Geometry: see drawing. Coordinates: mm, zero at the bounding-box minimum. A direction names the side the tool comes from. Coordinates: 2 decimals unless noted, no trailing zeros. Write each loop counter-clockwise with the first axis right and the second up, starting at its lowest first coordinate (ties: lowest second). Pieces come first, ordered by that corner, then holes. Notation, with made-up numbers: (-25.5, 61.25) - (-11.5, 61.25) arc R25 ccw to (-11.5, 96.25) - close; hole circle Ø11 at (24, 67.25). An arc over 180 degrees is marked (long way). Use a Markdown table: item, result. Add a question column.
Q1. Section query A-A (z = 4). Return the cut outline in (x, y).
Q2. Set-up query: the marked faces 1, 2 and 3. Return all of +Z, -Z, +X, -X, +Y, -Y with unobstructed straight access to the full face (end or side cutting, diameter ignored); none if empty.
Q3. Section query B-B (x = 28.5). Return the cut outline in (y, z).
Q4. Pin query (flat end, axial travel): P1, Ø5, axis at x = 24.5, y = 9.5, coming from the -Z side; P2, Ø8, axis at y = 10.5, z = 8, coming from the -X side; P3, Ø16, axis at x = 19.5, z = 27.5, coming from the +Y side. Return the tip coordinate at first contact, or that it passes through.
Q5. Section query C-C (x = 44). Return the cut outline in (y, z).
Q6. Section query D-D (z = 30). Return the cut outline in (x, y), then the cut area to 3 significant figures.
Q7. Mould query, pull axis Z, two halves, no side actions, for the marked faces 4, 5, 6 and 7. Classes: released by +Z, released by -Z, zero draft, split by the parting line, or undercut.
Q8. Material intervals for probe 1 along Y at (x, z) = (24, 18); probe 2 along X at (y, z) = (6, 23.5); probe 3 along Z at (x, y) = (64, 21.25), sorted ascending. Write a range as from..to.
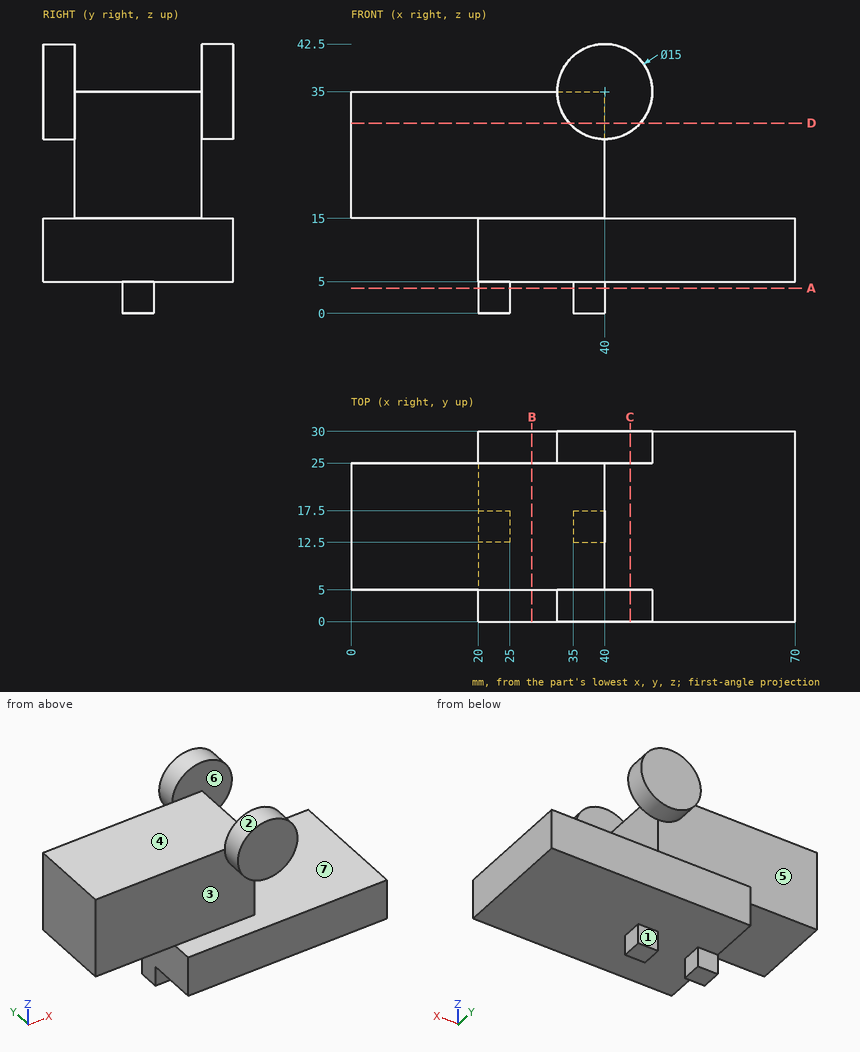
Values follow:
| question | item | result |
|---|---|---|
| 1 | outline | (20, 12.5) - (25, 12.5) - (25, 17.5) - (20, 17.5) - close; (35, 12.5) - (40, 12.5) - (40, 17.5) - (35, 17.5) - close |
| 2 | face 1 | -Z, +X, -X, +Y |
| 2 | face 2 | -Y |
| 2 | face 3 | -X, -Y |
| 3 | outline | (0, 5) - (30, 5) - (30, 15) - (25, 15) - (25, 35) - (5, 35) - (5, 15) - (0, 15) - close |
| 4 | P1 | z = 5 |
| 4 | P2 | x = 20 |
| 4 | P3 | y = 25 |
| 5 | outline | (0, 5) - (30, 5) - (30, 15) - (0, 15) - close; (0, 28.66) - (5, 28.66) - (5, 41.34) - (0, 41.34) - close; (25, 28.66) - (30, 28.66) - (30, 41.34) - (25, 41.34) - close |
| 6 | outline | (0, 5) - (34.41, 5) - (34.41, 0) - (45.59, 0) - (45.59, 5) - (40, 5) - (40, 25) - (45.59, 25) - (45.59, 30) - (34.41, 30) - (34.41, 25) - (0, 25) - close |
| 6 | area | 912 mm2 |
| 7 | face 4 | released by +Z |
| 7 | face 5 | undercut |
| 7 | face 6 | zero draft |
| 7 | face 7 | undercut |
| 8 | probe 1 | 5..25 |
| 8 | probe 2 | 0..40 |
| 8 | probe 3 | 5..15 |
